from build123d import *

# Parameters (mm, degrees)
SKETCH3_R          = 1.5
CUT_EXTRUDE2_DEPTH = 13


with BuildPart() as part:
    # Sketch1 → Revolve1 (revolve)
    with BuildSketch(Plane.XY, mode=Mode.PRIVATE) as revolve1_sk:
        with BuildLine():
            Line((0, 0), (0, 27))
            ThreePointArc((0, 27), (9.211074802, 24.939349426), (16.666049883, 19.150262594))
            ThreePointArc((16.666049883, 19.150262594), (8.466959251, 13.685208076), (10.355749103, 4.014407645))
            ThreePointArc((10.355749103, 4.014407645), (12.789115338, 1.999736062), (15.829018223, 1.139990011))
            ThreePointArc((15.829018223, 1.139990011), (16.650608773, 0.812513272), (17, 0))
            Line((17, 0), (0, 0))
        make_face()
    revolve(revolve1_sk.sketch.rotate(Axis((0, 0, 0), (0, 1, 0)), 90), axis=Axis((0, 0, 0), (0, 1, 0)))

    # Sketch3 → Cut-Extrude2 (cut)
    with BuildSketch(Plane.XZ):
        with Locations(Location((0, 0, 0), (0, 0, 270))):
            Circle(SKETCH3_R)
    extrude(amount=-CUT_EXTRUDE2_DEPTH, mode=Mode.SUBTRACT)


solid = part.part
Model file for the job. Use its own axes, mm. Give positions to 0.01 mm unless a question says otherwise; leave off trailing zeros. Loops run counter-clockwise (first coordinate to the right, second up) from the corner with the lowest first, then second, coordinate; pieces in that order, holes last.
1) Wall check: line 1 (Y direction, x = 6, z = -9.5); line 2 (Y direction, x = -2, z = 15); line 3 (Z direction, x = 9.5, y = 21.75). Give the ranges that are in metal, low to high.
2) Saw through at A-A (z = 0). Write the cut outline in (x, y), plus the area to 3 significant figures.
3) Pull direction Z, two halves, no side cores. Call faces 1 (the flat face through (0, 13, 0)), 2 (the cylindrical face through (0.45, 6.41, -1.43)), 3 (the flat face through (0, 0, -4)): +Z half, -Z half, draft (parallel to the pull), parting line (faces both ways), or undercut.
4) Saw through at C-C (y = 4.75). Write the cut outline in (x, z), plus the area to 3 significant figures.
5) Saw through at D-D (y = 17.5). Write the cut outline in (x, z), plus the area to 3 significant figures.
6) Flat gauge pins, fed straight in: pin 1 Ø1.5 at (x, z) = (0.5, 0) entering from -Y; pin 2 Ø6 at (x, z) = (5, -4.5) entering from +Y; pin 3 Ø1.5 at (x, y) = (-6.5, 10) entering from -Z. Where does each tip first touch, or does it go through?
7) Saw through at B-B (x = 0). Write the cut outline in (y, z), plus the area to 3 significant figures.
Answer block:
1. line 1: y = 0 to 3.08, 17.3 to 23.85
1. line 2: y = 0 to 1.22, 19.02 to 20.82
1. line 3: z = -10.45 to 10.45
2. outline: (-17, 0) - (-1.5, 0) - (-1.5, 13) - (1.5, 13) - (1.5, 0) - (17, 0) arc R1.16 ccw to (15.83, 1.14) arc R7.65 cw to (10.36, 4.01) arc R8.88 cw to (16.67, 19.15) arc R21.62 ccw to (-16.67, 19.15) arc R8.88 cw to (-10.36, 4.01) arc R7.65 cw to (-15.83, 1.14) arc R1.16 ccw to start
2. area: 530 mm2
3. face 1: undercut
3. face 2: undercut
3. face 3: draft
4. outline: circle Ø19.41 at (0, 0); hole circle Ø3 at (0, 0)
4. area: 289 mm2
5. outline: circle Ø23.02 at (0, 0)
5. area: 416 mm2
6. pin 1: stops at y = 13
6. pin 2: stops at y = 26.68
6. pin 3: stops at z = -5.25
7. outline: (0, -17) arc R1.16 ccw to (1.14, -15.83) arc R7.65 cw to (4.01, -10.36) arc R8.88 cw to (19.15, -16.67) arc R21.62 ccw to (19.15, 16.67) arc R8.88 cw to (4.01, 10.36) arc R7.65 cw to (1.14, 15.83) arc R1.16 ccw to (0, 17) - (0, 1.5) - (13, 1.5) - (13, -1.5) - (0, -1.5) - close
7. area: 530 mm2
